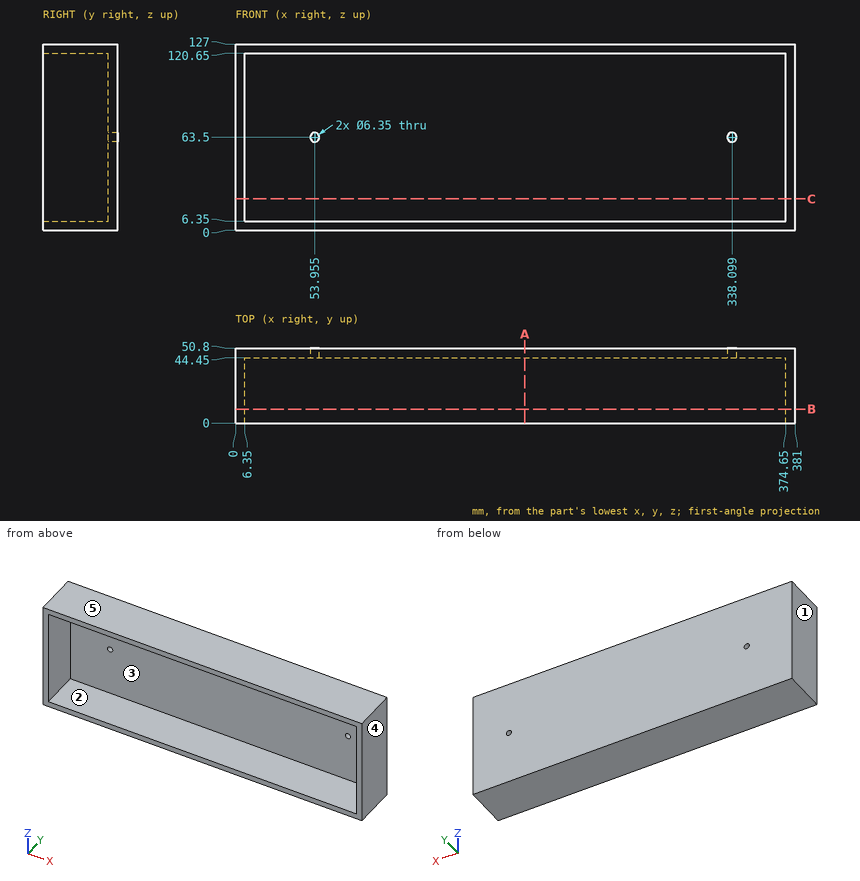
Here's the drawing with two shaded views (mm, measured from the low corner). I have some questions. A direction names the side the tool comes from. Round coordinates to 2 decimals unless told otherwise and drop trailing zeros. Loops run counter-clockwise (first coordinate to the right, second up) from the corner with the lowest first, then second, coordinate; pieces in that order, holes last.
1. If I drill on probe 1 along X at (y, z) = (12, 49); probe 2 along Z at (x, y) = (217, 33.5); probe 3 along Y at (x, z) = (97, 102), over which ranges is the centre line in solid material (lowest first)?
Answers:
probe 1: x = 0 to 6.35, 374.65 to 381
probe 2: z = 0 to 6.35, 120.65 to 127
probe 3: y = 44.45 to 50.8
2. Will these pins go through, and if not, where does the flat tip stop? pin 1 (4 mm diameter, centred on x = 338.1, z = 63.5, fed in from +Y); pin 2 (8.5 mm diameter, centred on x = 53.96, z = 63.5, fed in from -Y); pin 3 (10 mm diameter, centred on y = 20.5, z = 62.5, fed in from -X).
Answers:
pin 1: passes through
pin 2: stops at y = 44.45
pin 3: stops at x = 0
3. Thinking about a two-plate mould opening in Z: for the marked faces 3, 4 and 5, which applies, released by +Z, released by -Z, zero draft, split by the parting line, or undercut?
Answers:
face 3: undercut
face 4: zero draft
face 5: released by +Z
4. Suppose I cut it at B-B, the plane y = 9.5. Please give me the cut outline in (x, z).
Answers:
outline: (0, 0) - (381, 0) - (381, 127) - (0, 127) - close; hole (6.35, 6.35) - (374.65, 6.35) - (374.65, 120.65) - (6.35, 120.65) - close
5. Suppose I cut it at A-A, the plane x = 197. Please give me the cut outline in (y, z), and give its area (3 significant figures).
Answers:
outline: (0, 0) - (50.8, 0) - (50.8, 127) - (0, 127) - (0, 120.65) - (44.45, 120.65) - (44.45, 6.35) - (0, 6.35) - close
area: 1,370 mm2
6. Suppose I cut it at C-C, the plane z = 21.5. Please give me the cut outline in (x, y), and give its area (3 significant figures).
Answers:
outline: (0, 0) - (6.35, 0) - (6.35, 44.45) - (374.65, 44.45) - (374.65, 0) - (381, 0) - (381, 50.8) - (0, 50.8) - close
area: 2,980 mm2
7. For the marked faces 1 and 2, which set-ups out of +Z, -Z, +X, -X, +Y, -Y let a thin tool reach every point of the face, with its end or its side?
Answers:
face 1: +Z, -Z, -X, +Y, -Y
face 2: -Y
